Study the drawing (mm; zero at the part's minimum x, y, z) and answer. A direction names the side the tool comes from. Coordinates: 2 decimals unless noted, no trailing zeros. Write each loop counter-clockwise with the first axis right and the second up, starting at its lowest first coordinate (ties: lowest second). Pieces come first, ordered by that corner, then holes. Notation, with made-up numbers: (71.5, -15) -> (96.5, -15) arc R15 cw to (96.5, -9) -> close; hole circle Ø3 at (-30, 57.25). An arc over 180 degrees is marked (long way). Answer in a Markdown table with one row per item. Add a question column.
Item 1: Section B-B on z = 1.75 is taken. Write down the section's boundary in (x, y), then the cut area to 3 significant figures.
Item 2: Section A-A on x = 8 is taken. Write down the section's boundary in (y, z).
Item 3: Given pin 1 Ø1 at (x, y) = (11, 3.5) entering from -Z; pin 2 Ø4 at (x, y) = (12, 3) entering from -Z; pin 3 Ø4 at (x, z) = (8, 8) entering from -Y; pin 4 Ø1 at (x, y) = (7, 12) entering from +Z, each flat-ended and moving along its own axis, determine where each tip first touches the part or whether it passes through.
Item 4: For a pull along Y with two mould halves and no side action, classify the marked faces 1, 2, 3 and 4 as +Y half, -Y half, draft (parallel to the pull), parting line (faces both ways), or undercut.
Item 5: Section C-C on y = 13.5 is taken. Write down the section's boundary in (x, z), then the cut area to 3 significant figures.
Item 6: Section D-D on x = 11.5 is taken. Write down the section's boundary in (y, z), then the cut area to 3 significant figures.
Item 7: Straight lines are drawn through the part: line 1 (X direction, y = 5.5, z = 8); line 2 (Y direction, x = 2, z = 11.5); line 3 (X direction, y = 10.5, z = 8). For each, find the intervals that lie inside material, in ascending order. Write a range as from..to.
Item 8: Which of the six approach directions +Z, -Z, +X, -X, +Y, -Y give full straight-line access (tool end or side, diameter ignored) to the marked faces 5 and 6?
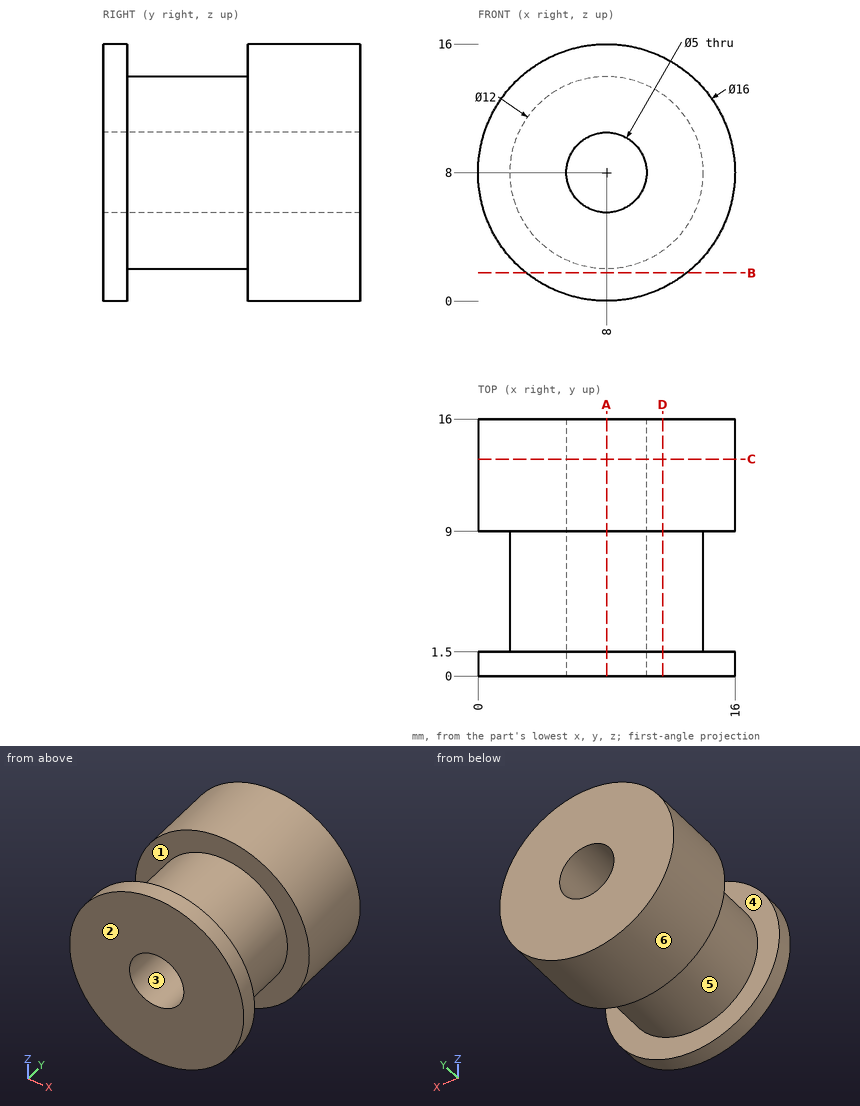
Results below:
| question | item | result |
|---|---|---|
| 1 | outline | (3.01, 0) -> (12.99, 0) -> (12.99, 1.5) -> (3.01, 1.5) -> close; (3.01, 9) -> (12.99, 9) -> (12.99, 16) -> (3.01, 16) -> close |
| 1 | area | 84.9 mm2 |
| 2 | outline | (0, 0) -> (1.5, 0) -> (1.5, 2) -> (9, 2) -> (9, 0) -> (16, 0) -> (16, 5.5) -> (0, 5.5) -> close; (0, 10.5) -> (16, 10.5) -> (16, 16) -> (9, 16) -> (9, 14) -> (1.5, 14) -> (1.5, 16) -> (0, 16) -> close |
| 3 | pin 1 | stops at z = 2.55 |
| 3 | pin 2 | stops at z = 0.46 |
| 3 | pin 3 | passes through |
| 3 | pin 4 | stops at z = 15.98 |
| 4 | face 1 | undercut |
| 4 | face 2 | -Y half |
| 4 | face 3 | draft |
| 4 | face 4 | undercut |
| 5 | outline | circle Ø16 at (8, 8); hole circle Ø5 at (8, 8) |
| 5 | area | 181 mm2 |
| 6 | outline | (0, 0.81) -> (1.5, 0.81) -> (1.5, 3.13) -> (9, 3.13) -> (9, 0.81) -> (16, 0.81) -> (16, 15.19) -> (9, 15.19) -> (9, 12.87) -> (1.5, 12.87) -> (1.5, 15.19) -> (0, 15.19) -> close |
| 6 | area | 195 mm2 |
| 7 | line 1 | x = 2..5.5, 10.5..14 |
| 7 | line 2 | y = 0..1.5, 9..16 |
| 7 | line 3 | x = 0..5.5, 10.5..16 |
| 8 | face 5 | none |
| 8 | face 6 | +Y, -Y |
